Part model, mm, in its own coordinate system. Face numbers are marked on the shaded views. A direction names the side the tool comes from. Give positions to 0.01 mm unless a question says otherwise; leave off trailing zeros. Loops run counter-clockwise (first coordinate to the right, second up) from the corner with the lowest first, then second, coordinate; pieces in that order, holes last. Notation, with made-up numbers: (-20, -39) -> (8, -39) arc R28 cw to (8, -21) -> close; hole circle Ø6 at (-0.5, 38.25). An arc over 180 degrees is marked (long way). Write item = value, one per line.
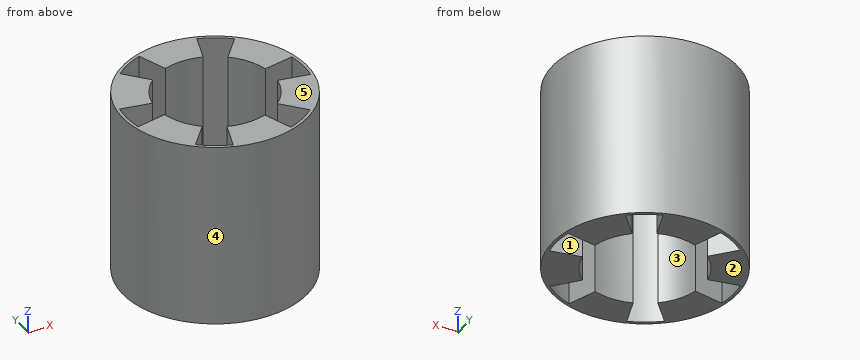
from build123d import *

# Parameters (mm, degrees)
SKETCH4_R           = 30
BOSS_EXTRUDE2_DEPTH = 60
CUT_EXTRUDE1_DEPTH  = 74.484692283


with BuildPart() as part:
    # Sketch4 → Boss-Extrude2 (new body)
    with BuildSketch(Plane.XY):
        Circle(SKETCH4_R)
    extrude(amount=BOSS_EXTRUDE2_DEPTH)

    # Sketch5 → Cut-Extrude1 (cut, through all)
    with BuildSketch(Plane(origin=(0, 0, 0), x_dir=(-1, 0, 0), z_dir=(0, 0, -1))):
        with BuildLine():
            Line((-6.249262611, 17.942873706), (-9.538348196, 27.386491445))
            ThreePointArc((-9.538348196, 27.386491445), (-14.5, 25.11473671), (-18.948223214, 21.953697571))
            Line((-18.948223214, 21.953697571), (-12.41435314, 14.383457029))
            ThreePointArc((-12.41435314, 14.383457029), (-16.454482672, 9.5), (-18.663615752, 3.559416677))
            Line((-18.663615752, 3.559416677), (-28.48657141, 5.432793875))
            ThreePointArc((-28.48657141, 5.432793875), (-29, 0), (-28.48657141, -5.432793875))
            Line((-28.48657141, -5.432793875), (-18.663615752, -3.559416677))
            ThreePointArc((-18.663615752, -3.559416677), (-16.454482672, -9.5), (-12.41435314, -14.383457029))
            Line((-12.41435314, -14.383457029), (-18.948223214, -21.953697571))
            ThreePointArc((-18.948223214, -21.953697571), (-14.5, -25.11473671), (-9.538348196, -27.386491445))
            Line((-9.538348196, -27.386491445), (-6.249262611, -17.942873706))
            ThreePointArc((-6.249262611, -17.942873706), (0, -19), (6.249262611, -17.942873706))
            Line((6.249262611, -17.942873706), (9.538348196, -27.386491445))
            ThreePointArc((9.538348196, -27.386491445), (14.5, -25.11473671), (18.948223214, -21.953697571))
            Line((18.948223214, -21.953697571), (12.41435314, -14.383457029))
            ThreePointArc((12.41435314, -14.383457029), (16.454482672, -9.5), (18.663615752, -3.559416677))
            Line((18.663615752, -3.559416677), (28.48657141, -5.432793875))
            ThreePointArc((28.48657141, -5.432793875), (29, 0), (28.48657141, 5.432793875))
            Line((28.48657141, 5.432793875), (18.663615752, 3.559416677))
            ThreePointArc((18.663615752, 3.559416677), (16.454482672, 9.5), (12.41435314, 14.383457029))
            Line((12.41435314, 14.383457029), (18.948223214, 21.953697571))
            ThreePointArc((18.948223214, 21.953697571), (14.5, 25.11473671), (9.538348196, 27.386491445))
            Line((9.538348196, 27.386491445), (6.249262611, 17.942873706))
            ThreePointArc((6.249262611, 17.942873706), (0, 19), (-6.249262611, 17.942873706))
        make_face()
    extrude(amount=-CUT_EXTRUDE1_DEPTH, mode=Mode.SUBTRACT)


solid = part.part
1) Drill centre lines: line 1 along X through (y, z) = (-0.5, 3.5); line 2 along X through (y, z) = (-25, 18.5); line 3 along Y through (x, z) = (-14.5, 23). Where is each one in solid material? Low to high. Write a range as [from, to].
Resolved:
line_1 = [-30, -29], [29, 30]
line_2 = [-16.58, -14.7], [-8.71, 8.71], [14.7, 16.58]
line_3 = [-26.26, -25.11], [-16.8, -12.28], [12.28, 16.8], [25.11, 26.26]
2) Which spindle directions (+Z, -Z, +X, -X, +Y, -Y) get a long thin tool onto all of the face, cutting with end or side? Do the marked faces 1 and 2. Say none if no direction does.
Resolved:
face_1 = +Z, -Z
face_2 = -Z, +X, -X, +Y, -Y
3) Slice it at D-D, the plane y = 24.5. List the corners of the cut face in (x, z).
Resolved:
outline = (-17.31, 0) -> (-15.52, 0) -> (-15.52, 60) -> (-17.31, 60) -> close; (-8.53, 0) -> (8.53, 0) -> (8.53, 60) -> (-8.53, 60) -> close; (15.52, 0) -> (17.31, 0) -> (17.31, 60) -> (15.52, 60) -> close
4) Slice it at C-C, the plane y = 0. List the corners of the cut face in (x, z), and give its area (3 significant figures).
Resolved:
outline = (-30, 0) -> (-29, 0) -> (-29, 60) -> (-30, 60) -> close; (29, 0) -> (30, 0) -> (30, 60) -> (29, 60) -> close
area = 120 mm²
5) Pull direction X, two halves, no side cores. Call the marked faces 3, 4 and 5: pulls with the +X half, pulls with the -X half, needs draft (parallel to the pull), parting line crosses it, or undercut.
Resolved:
face_3 = undercut
face_4 = parting line crosses it
face_5 = needs draft
6) Slice it at A-A, the plane x = 0. List the corners of the cut face in (y, z), and give its area (3 significant figures).
Resolved:
outline = (-30, 0) -> (-19, 0) -> (-19, 60) -> (-30, 60) -> close; (19, 0) -> (30, 0) -> (30, 60) -> (19, 60) -> close
area = 1,320 mm²
7) Slice it at B-B, the plane z = 46. List the corners of the cut face in (x, y), and give its area (3 significant figures).
Resolved:
outline = circle Ø60 at (0, 0); hole (-28.49, -5.43) -> (-18.66, -3.56) arc R19 ccw to (-12.41, -14.38) -> (-18.95, -21.95) arc R29 ccw to (-9.54, -27.39) -> (-6.25, -17.94) arc R19 ccw to (6.25, -17.94) -> (9.54, -27.39) arc R29 ccw to (18.95, -21.95) -> (12.41, -14.38) arc R19 ccw to (18.66, -3.56) -> (28.49, -5.43) arc R29 ccw to (28.49, 5.43) -> (18.66, 3.56) arc R19 ccw to (12.41, 14.38) -> (18.95, 21.95) arc R29 ccw to (9.54, 27.39) -> (6.25, 17.94) arc R19 ccw to (-6.25, 17.94) -> (-9.54, 27.39) arc R29 ccw to (-18.95, 21.95) -> (-12.41, 14.38) arc R19 ccw to (-18.66, 3.56) -> (-28.49, 5.43) arc R29 ccw to start
area = 1,150 mm²
8) Drop flat-ended pins along their axis: P1, Ø5, axis at x = 5.5, z = 35.5, coming from the -Y side; P2, Ø1.5, axis at y = 14.5, z = 31.5, coming from the -X side; P3, Ø8, axis at x = 1, z = 32.5, coming from the +Y side; P4, Ø6, axis at x = 10, y = -19, coming from the +Z side. Give the stop position or say it passes through.
Resolved:
P1 = -29.85
P2 = -26.66
P3 = 30
P4 = through
